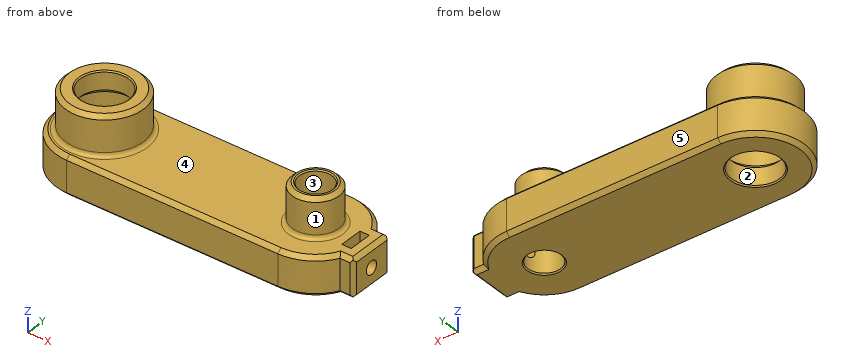
Autodesk Fusion 360 part; units mm, degrees
sketch "Esquisse1" plane through (0, 0, 0) normal (0, 0, 1) x (1, 0, 0)
  circle A0 centre (-55.5807, 0.978) radius 6.2
  circle A1 centre (-1.1807, 0.978) radius 4.2
  line L0 (-55.5807, 13.478) -> (-1.1807, 13.478)
  line L1 (-1.1807, 13.478) -> (-1.1807, -11.522) construction
  line L2 (-1.1807, -11.522) -> (-55.5807, -11.522)
  line L3 (-55.5807, -11.522) -> (-55.5807, 13.478) construction
  arc A2 (-55.5807, 13.478) -> (-55.5807, -11.522) centre (-55.5807, 0.978) ccw
  line L4 (9.7852, -5.022) -> (13.2852, -5.022)
  line L5 (13.2852, -5.022) -> (13.2852, 6.978)
  line L6 (13.2852, 6.978) -> (9.7852, 6.978)
  arc A3 (-1.1807, -11.522) -> (9.7852, -5.022) centre (-1.1807, 0.978) ccw
  arc A4 (9.7852, 6.978) -> (-1.1807, 13.478) centre (-1.1807, 0.978) ccw
  dimension "d1" = 54.4
  dimension "d2" = 12.4
  dimension "d3" = 8.4
  dimension "d4" = 25
  dimension "d5" = 12.5
  dimension "d7" = 12
  dimension "d8" = 3.5
extrude "Extrusion1" add sketch "Esquisse1" along normal blind 10
sketch "Esquisse2" plane through (0, 0, 10) normal (0, 0, 1) x (-1, 0, 0)
  circle A0 centre (55.5807, -0.978) radius 6.2
  circle A1 centre (1.1807, -0.978) radius 4.2
  arc A2 (1.1807, 11.522) -> (-9.7852, 5.022) centre (1.1807, -0.978) ccw
  line L0 (-9.7852, 5.022) -> (-13.2852, 5.022)
  line L1 (-13.2852, 5.022) -> (-13.2852, -6.978)
  line L2 (-13.2852, -6.978) -> (-9.7852, -6.978)
  arc A3 (-9.7852, -6.978) -> (1.1807, -13.478) centre (1.1807, -0.978) ccw
  line L3 (1.1807, -13.478) -> (55.5807, -13.478)
  arc A4 (55.5807, -13.478) -> (55.5807, 11.522) centre (55.5807, -0.978) ccw
  line L4 (55.5807, 11.522) -> (1.1807, 11.522)
  circle A5 centre (55.5807, -0.978) radius 10
  circle A6 centre (1.1807, -0.978) radius 6
  circle A7 centre (55.5807, -0.978) radius 7.5
  dimension "d11" = 20
  dimension "d12" = 12
  dimension "d32" = 15
extrude "Extrusion4" add sketch "Esquisse2" along normal blind 10 contours A5 | A6 | A7
extrude "Extrusion5" cut sketch "Esquisse2" along normal mid plane 8 contours A7
chamfer "Chanfrein3" distance 1.3 angle 45 2 edges at (-61.3611, -1.264, 6) (-61.3611, 3.2201, 14)
ref_plane "Plan de construction2" through (10.2852, 0.978, 5) normal (1, 0, 0) x (0, 1, 0)
sketch "Esquisse3" plane through (10.2852, 0, 0) normal (1, 0, 0) x (0, 1, 0)
  line L0 (-5.022, 0) -> (6.978, 0)
  line L1 (6.978, 0) -> (6.978, 10)
  line L2 (6.978, 10) -> (-5.022, 10)
  line L3 (-5.022, 10) -> (-5.022, 0)
  line L4 (-2.022, 10) -> (3.978, 10)
  line L5 (3.978, 10) -> (3.978, 5)
  line L6 (3.978, 5) -> (-2.022, 5) construction
  line L7 (-2.022, 5) -> (-2.022, 10)
  line L8 (0.978, 5) -> (0.978, 1.9) construction
  line L9 (-2.022, 6.7321) -> (-2.022, 3.2679)
  line L10 (-2.022, 3.2679) -> (0.978, 1.5359)
  line L11 (0.978, 1.5359) -> (3.978, 3.2679)
  line L12 (3.978, 3.2679) -> (3.978, 6.7321)
  point P0 (0.978, 5)
  dimension "d15" = 3.1
  dimension "d16" = 5
  dimension "d17" = 6
  dimension "d18" = 12
  dimension "d19" = 3
extrude "Extrusion3" cut sketch "Esquisse3" against normal blind 2.4 contours L2 L4 L5 L7 L9 L10 L11 L12
hole "Perçage1" at (13.2852, 0.8569, 5) direction (-1, 0, 0) diameter 3.4 depth 11 tip angle 180
chamfer "Chanfrein1" distance 1 angle 45 16 edges at (5.1931, -9.7749, 10) (5.1931, 11.7309, 10) (-28.3807, 13.478, 10) (-68.0807, 0.978, 10) (-28.3807, -11.522, 10) (-28.3807, -11.522, 0) (-68.0807, 0.978, 0) (-28.3807, 13.478, 0) (5.1931, 11.7309, 0) (5.1931, -9.7749, 0) (11.5352, -5.022, 0) (11.5352, -5.022, 10) (13.2852, 0.978, 0) (13.2852, 0.978, 10) (11.5352, 6.978, 10) (11.5352, 6.978, 0)
chamfer "Chanfrein2" distance 1 angle 45 2 edges at (13.2852, 6.978, 5) (13.2852, -5.022, 5)
chamfer "Chanfrein4" distance 0.3 angle 45 4 edges at (-49.8002, -1.264, 20) (-61.3611, 3.2201, 0) (2.7351, -0.5407, 20) (-5.0964, 2.4968, 0)
fillet "Congé2" radius 1 2 edges at (-46.2574, -2.6381, 10) (4.4133, -1.1917, 10)
chamfer "Chanfrein5" distance 1 angle 45 2 edges at (4.4133, 3.1477, 20) (-46.2574, 4.5942, 20)
equation "d5 = d4 / 2"
equation "d19 = ( d18 - d17 ) / 2"
equation "d30 = d9"
Verification items for the finished model (mm, model axes). Face numbers are marked on the shaded views. A direction names the side the tool comes from. Give positions to 0.01 mm unless a question says otherwise; leave off trailing zeros. Loops run counter-clockwise (first coordinate to the right, second up) from the corner with the lowest first, then second, coordinate; pieces in that order, holes last. Notation, with made-up numbers: (11, -24.5) - (16, -24.5) arc R18 ccw to (16, -8.5) - close; hole circle Ø9 at (76.25, 86.5). An arc over 180 degrees is marked (long way). Write item = value, one per line. Start each with the question number.
Q1. Depth check by flat-ended pin: P1, Ø4, axis at x = -25, y = -9, coming from the +Z side; P2, Ø4, axis at y = 5.5, z = 11.5, coming from the -X side; P3, Ø1.2, axis at x = 11.5, z = 3.5, coming from the +Y side; P4, Ø7.5, axis at x = -1.18, y = 0.98, coming from the -Z side. Enter the tip coordinate at first touch or a pass-through.
Q2. Cross-section at A-A, the plane x = -43. Enter the section's corners in (y, z), and give its area (3 significant figures).
Q3. Thickness scan on line 1 (X direction, y = 1.25, z = 1); line 2 (Y direction, x = 11.4, z = 5); line 3 (X direction, y = -0.5, z = 19.25). Record the ranges inside material, lowest first.
Q4. Tool access check on the marked faces 1 and 2. Record the directions out of +Z, -Z, +X, -X, +Y, -Y that give a thin tool (end or side, any length) a straight path to the whole face; none if there is none.
Q5. Mould release check, pull along Y, two halves, no side actions. Record for the marked faces 3, 4 and 5: released by +Y, released by -Y, zero draft, split by the parting line, or undercut.
Answer key:
q1.P1 = 10
q1.P2 = -66.82
q1.P3 = 6.98
q1.P4 = through
q2.outline = (-11.52, 1) - (-10.52, 0) - (12.48, 0) - (13.48, 1) - (13.48, 9) - (12.48, 10) - (-10.52, 10) - (-11.52, 9) - close
q2.area = 248 mm^2
q3.line_1 = -68.08 to -61.77, -49.39 to -5.37, 3.01 to 13.29
q3.line_2 = -5.02 to -0.84, 2.56 to 6.98
q3.line_3 = -65.22 to -61.6, -49.56 to -45.94, -6.74 to -5.11, 2.75 to 4.38
q4.face_1 = +Z
q4.face_2 = +Z, -Z
q5.face_3 = undercut
q5.face_4 = zero draft
q5.face_5 = released by +Y
